```python
from build123d import *

# Parameters (mm, degrees)
CROQUIS1_W                 = 1000
CROQUIS1_H                 = 2000
SALIENTE_EXTRUIR2_DEPTH    = 40
CROQUIS2_W                 = 940
CROQUIS2_H                 = 1940
CORTAR_EXTRUIR1_DEPTH      = 30
CORTAR_EXTRUIR2_DEPTH      = 495
CORTAR_EXTRUIR2_DEPTH_BACK = 495
CROQUIS3_W                 = 25
CROQUIS3_H                 = 1990
CROQUIS4_W                 = 970
CROQUIS4_H                 = 1970
CORTAR_EXTRUIR3_DEPTH      = 5


with BuildPart() as part:
    # Croquis1 → Saliente-Extruir2 (new body)
    with BuildSketch(Plane.XY):
        Rectangle(CROQUIS1_W, CROQUIS1_H)
    extrude(amount=SALIENTE_EXTRUIR2_DEPTH)

    # Croquis2 → Cortar-Extruir1 (cut)
    with BuildSketch(Plane(origin=(0, 0, 0), x_dir=(-1, 0, 0), z_dir=(0, 0, -1))):
        Rectangle(CROQUIS2_W, CROQUIS2_H)
    extrude(amount=-CORTAR_EXTRUIR1_DEPTH, mode=Mode.SUBTRACT)

    # Croquis3 → Cortar-Extruir2 (cut, two sides: drawn at the far end of the back side and taken through both)
    with BuildSketch(Plane(origin=(0, 0, 0), x_dir=(0, 0, -1), z_dir=(1, 0, 0)).offset(-CORTAR_EXTRUIR2_DEPTH_BACK)):
        with Locations((-17.5, 0)):
            Rectangle(CROQUIS3_W, CROQUIS3_H)
    extrude(amount=CORTAR_EXTRUIR2_DEPTH + CORTAR_EXTRUIR2_DEPTH_BACK, mode=Mode.SUBTRACT)

    # Croquis4 → Cortar-Extruir3 (cut)
    with BuildSketch(Plane.XY.offset(40)):
        Rectangle(CROQUIS4_W, CROQUIS4_H)
    extrude(amount=-CORTAR_EXTRUIR3_DEPTH, mode=Mode.SUBTRACT)


solid = part.part
```
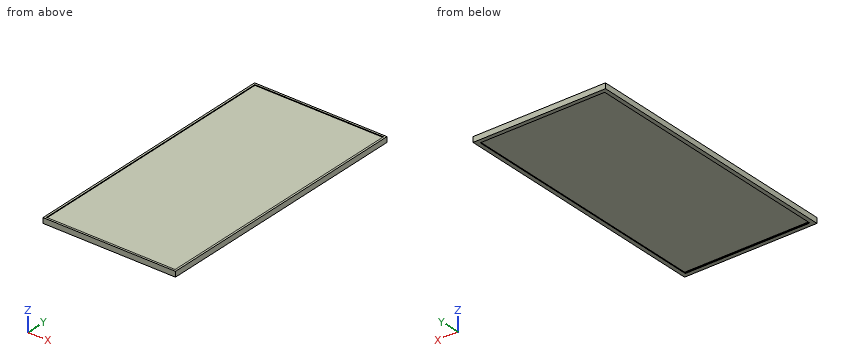
Geometry: final body of the model. Coordinates: model frame, mm. Coordinates: 2 decimals unless noted, no trailing zeros. Order: outer loops, then holes, each group sorted by start corner. A loop starts at its lowest first (then second) coordinate and runs counter-clockwise, first axis right, second up. Notation, with made-up numbers: (41.25, 72) - (54.25, 72) arc R28 ccw to (54.25, 92) - close; hole circle Ø4 at (34, -22). An arc over 180 degrees is marked (long way). Return JSON: item names as keys, results as strings. Group by question number.
1. Cut plane B-B (y = -657). Output: boundary loops of the cut face in (x, z).
2. Cut plane C-C (z = 15). Output: boundary loops of the cut face in (x, y), plus the area to 3 significant figures.
3. Cut plane A-A (x = -413). Output: boundary loops of the cut face in (y, z), plus the area to 3 significant figures.
4. Material intervals for line 1 along Y through (x, z) = (99.5, 19.5); line 2 along X through (y, z) = (-282, 16.5); line 3 along Y through (x, z) = (354, 4), sorted ascending. Write a range as [from, to].
5. Pin query (flat end, axial travel): pin 1 (8 mm diameter, centred on x = 9, y = 757, fed in from +Z); pin 2 (1 mm diameter, centred on x = -153.5, y = -135, fed in from -Z). Return the tip coordinate at first contact, or that it passes through.
Resolved:
{
 "1": {"outline": "(-500, 0) - (-470, 0) - (-470, 5) - (-495, 5) - (-495, 30) - (495, 30) - (495, 5) - (470, 5) - (470, 0) - (500, 0) - (500, 40) - (485, 40) - (485, 35) - (-485, 35) - (-485, 40) - (-500, 40) - close"},
 "2": {"outline": "(-500, -1000) - (500, -1000) - (500, 1000) - (-500, 1000) - close; hole (-495, -995) - (495, -995) - (495, 995) - (-495, 995) - close", "area": "29,900 mm²"},
 "3": {"outline": "(-1000, 0) - (-970, 0) - (-970, 5) - (-995, 5) - (-995, 30) - (995, 30) - (995, 5) - (970, 5) - (970, 0) - (1000, 0) - (1000, 40) - (985, 40) - (985, 35) - (-985, 35) - (-985, 40) - (-1000, 40) - close", "area": "10,700 mm²"},
 "4": {"line 1": "y = [-1000, -995], [995, 1000]", "line 2": "x = [-500, -495], [495, 500]", "line 3": "y = [-1000, -970], [970, 1000]"},
 "5": {"pin 1": "stops at z = 35", "pin 2": "stops at z = 30"}
}
